Can you work these out from the model? Positions are in its coordinate system, mm. A direction names the side the tool comes from. Round coordinates to 2 decimals unless told otherwise and drop trailing zeros. Loops run counter-clockwise (first coordinate to the right, second up) from the corner with the lowest first, then second, coordinate; pieces in that order, holes last.
(1) Which directions (+Z, -Z, +X, -X, +Y, -Y) give clear straight access to the entire face, cutting with the end or side of a thin tool? Please do faces 1 (the face through (-42.922, -43.001, 6.439)), 2 (the face through (56, -31.75, 3)), 3 (the face through (42.922, -43.001, 9.569)).
(2) I want a section at A-A on z = 1.75. Write out the boundary of the cut face in (x, y) (3 decimals), plus the area to 3 significant figures.
(3) I want a section at D-D on y = -38. Write out the boundary of the cut face in (x, z).
(4) Thinking about a two-plate mould opening in X: for faces 4 (the face through (9, -44.45, 6)), 5 (the face through (44.45, -1, 6)), 6 (the face through (-28.547, 1.256, 6.439)), which applies, released by +X, released by -X, zero draft, split by the parting line, or undercut?
(5) Will these pins go through, and if not, where does the flat tip stop? pin 1 Ø1.5 at (y, z) = (-28, 10.5) entering from +X; pin 2 Ø5 at (x, z) = (54.5, 3.5) entering from +Y.
(6) I want a section at B-B on y = 0. Write out the boundary of the cut face in (x, z) (3 decimals).
(7) If I drill on line 1 along Y through (x, z) = (0, 8.75) (3 decimals); line 2 along Y through (x, z) = (57, 5.5); line 3 along X through (y, z) = (-7, 10), over which ranges is the centre line in solid material (lowest first)?
(8) I want a section at C-C on x = -4. Write out the boundary of the cut face in (y, z).
from build123d import *

# Parameters (mm, degrees)
F1_DEPTH = 12.7
F0_W     = 19.05
F0_H     = 12.7
F2_DEPTH = 6.35
F3_R     = 5.08
F4_R     = 5.08
F5_R     = 28.575
F6_DEPTH = 25.4


with BuildPart() as f1:
    # F0 (on Top) → F1 (new body)
    with BuildSketch(Plane.XY):
        Polygon((44.45, 44.45), (-44.45, 44.45), (-44.45, -44.45), (44.45, -44.45), (44.45, -31.75), align=None)
    extrude(amount=F1_DEPTH)

    # F0 (on Top) → F2 (join)
    with BuildSketch(Plane.XY):
        with Locations((53.975, -38.1)):
            Rectangle(F0_W, F0_H)
    extrude(amount=F2_DEPTH)

    # F3
    f3_edges = [f1.edges().sort_by_distance(p)[0] for p in [
        (-44.45, -44.45, 6.35),
        (-44.45, 44.45, 6.35),
        (44.45, 44.45, 6.35),
        (44.45, -31.75, 3.175),
    ]]
    fillet(f3_edges, radius=F3_R)

    # F4
    f4_edges = [f1.edges().sort_by_distance(p)[0] for p in [
        (44.45, -44.45, 9.525),
        (63.5, -44.45, 3.175),
    ]]
    fillet(f4_edges, radius=F4_R)

    # F5 (on face) → F6 (cut)
    with BuildSketch(Plane.XY.offset(12.7)):
        Circle(F5_R)
    extrude(amount=-F6_DEPTH, mode=Mode.SUBTRACT)


solid = f1.part
Filled sheet:
1. face 1: +Z, -Z, -X, -Y
1. face 2: +Z, -Z, +X, +Y
1. face 3: +Z, +X, -Y
2. outline: (-44.45, -39.37) arc R5.08 ccw to (-39.37, -44.45) - (58.42, -44.45) arc R5.08 ccw to (63.5, -39.37) - (63.5, -31.75) - (49.53, -31.75) arc R5.08 cw to (44.45, -26.67) - (44.45, 39.37) arc R5.08 ccw to (39.37, 44.45) - (-39.37, 44.45) arc R5.08 ccw to (-44.45, 39.37) - close; hole circle Ø57.15 at (0, 0)
2. area: 5,560 mm2
3. outline: (-44.45, 0) - (63.5, 0) - (63.5, 6.35) - (44.45, 6.35) - (44.45, 12.7) - (-44.45, 12.7) - close
4. face 4: zero draft
4. face 5: released by +X
4. face 6: undercut
5. pin 1: stops at x = 44.45
5. pin 2: stops at y = -31.75
6. outline: (-44.45, 0) - (-28.575, 0) - (-28.575, 12.7) - (-44.45, 12.7) - close; (28.575, 0) - (44.45, 0) - (44.45, 12.7) - (28.575, 12.7) - close
7. line 1: y = -44.45 to -28.575, 28.575 to 44.45
7. line 2: y = -44.45 to -31.75
7. line 3: x = -44.45 to -27.7, 27.7 to 44.45
8. outline: (-44.45, 0) - (-28.29, 0) - (-28.29, 12.7) - (-44.45, 12.7) - close; (28.29, 0) - (44.45, 0) - (44.45, 12.7) - (28.29, 12.7) - close
